Here's how the part is built. I have some questions about the finished solid (model axes, mm). A direction names the side the tool comes from. Coordinates: 2 decimals unless noted, no trailing zeros. Loops run counter-clockwise (first coordinate to the right, second up) from the corner with the lowest first, then second, coordinate; pieces in that order, holes last.
from build123d import *

# Parameters (mm, degrees)
F0_W     = 50.8
F0_H     = 50.8
F1_DEPTH = 254
F2_W     = 44.45
F2_H     = 44.45
F3_DEPTH = 254.001
F4_R     = 4.7625
F5_DEPTH = 50.801


with BuildPart() as f1:
    # F0 (on Top) → F1 (new body)
    with BuildSketch(Plane.XY):
        with Locations((25.4, 25.4)):
            Rectangle(F0_W, F0_H)
    extrude(amount=F1_DEPTH)

    # F2 (on face) → F3 (cut, through all)
    with BuildSketch(Plane.XY.offset(254)):
        with Locations((25.4, 25.4)):
            Rectangle(F2_W, F2_H)
    extrude(amount=-F3_DEPTH, mode=Mode.SUBTRACT)

    # F4 (on face) → F5 (cut, through all)
    with BuildSketch(Plane.YZ.offset(50.8)):
        with Locations((25.4, 12.7)):
            Circle(F4_R)
        with Locations((25.4, 38.1)):
            Circle(F4_R)
        with Locations((25.4, 63.5)):
            Circle(F4_R)
        with Locations((25.4, 88.9)):
            Circle(F4_R)
        with Locations((25.4, 114.3)):
            Circle(F4_R)
        with Locations((25.4, 139.7)):
            Circle(F4_R)
        with Locations((25.4, 165.1)):
            Circle(F4_R)
        with Locations((25.4, 190.5)):
            Circle(F4_R)
        with Locations((25.4, 215.9)):
            Circle(F4_R)
        with Locations((25.4, 241.3)):
            Circle(F4_R)
    extrude(amount=-F5_DEPTH, mode=Mode.SUBTRACT)


solid = f1.part
Q1. We'd pull the mould along Y, two halves only. Please class faces 1 (the flat face through (3, 26, 0)), 2 (the flat face through (47.625, 25, 129)), 3 (the flat face through (3.175, 25, 129)): pulls with the +Y half, pulls with the -Y half, needs draft (parallel to the pull), parting line crosses it, or undercut.
Q2. Suppose I cut it at A-A on y = 36. Write out the boundary of the cut face in (x, z) (3 decimals), and give its area (3 significant figures).
Q3. Please list where these lines run through material, in increasing order: probe 1 along Y at (x, z) = (31, 153) (3 decimals); probe 2 along Y at (x, z) = (2, 139).
Q4. Suppose I cut it at D-D on z = 54.5. Write out the boundary of the cut face in (x, y) (3 decimals), and give its area (3 significant figures).
Q5. For faces 4 (the cylindrical face through (49.23, 24.78, 119.02)), 5 (the flat face through (25, 47.625, 129)), which set-ups out of +Z, -Z, +X, -X, +Y, -Y let a thin tool reach every point of the face, with its end or its side?
Q6. Suppose I cut it at B-B on z = 165.1. Write out the boundary of the cut face in (x, y) (1 decimal), and give its area (3 significant figures).
Check values:
1. face 1: needs draft
1. face 2: undercut
1. face 3: undercut
2. outline: (0, 0) - (3.175, 0) - (3.175, 254) - (0, 254) - close; (47.625, 0) - (50.8, 0) - (50.8, 254) - (47.625, 254) - close
2. area: 1,610 mm2
3. probe 1: y = 0 to 3.175, 47.625 to 50.8
3. probe 2: y = 0 to 20.69, 30.11 to 50.8
4. outline: (0, 0) - (50.8, 0) - (50.8, 50.8) - (0, 50.8) - close; hole (3.175, 3.175) - (47.625, 3.175) - (47.625, 47.625) - (3.175, 47.625) - close
4. area: 605 mm2
5. face 4: +X, -X
5. face 5: +Z, -Z
6. outline: (0, 0) - (50.8, 0) - (50.8, 20.6) - (47.6, 20.6) - (47.6, 3.2) - (3.2, 3.2) - (3.2, 20.6) - (0, 20.6) - close; (0, 30.2) - (3.2, 30.2) - (3.2, 47.6) - (47.6, 47.6) - (47.6, 30.2) - (50.8, 30.2) - (50.8, 50.8) - (0, 50.8) - close
6. area: 544 mm2
